The listing builds one solid part. Answer for the finished solid, in the listing's coordinates (mm). A direction names the side the tool comes from. Round coordinates to 2 decimals unless told otherwise and drop trailing zeros. Write each loop counter-clockwise with the first axis right and the second up, starting at its lowest first coordinate (ties: lowest second). Pieces come first, ordered by that corner, then holes.
(1) Find the intervals of material crossed by probe 1 along X at (y, z) = (10.8, 0); probe 2 along Y at (x, z) = (0, 11.75) (3 decimals); probe 3 along X at (y, z) = (7, 2.5), in increasing order.
(2) A cutting plane is placed at C-C, the plane x = 17.5. Give the vertices of the cut face in (y, z).
(3) For faces 4 (the face through (0, 6, -20.41)), 5 (the face through (-0.116, 2.827, 7.888)), 6 (the face through (0, 9, -18)), determine the directions among +Z, -Z, +X, -X, +Y, -Y from which every point of the face is accessible in a straight line to the end or side of a thin tool.
(4) The mould has two halves that part along Y. Classify faces 1 (the face through (-2.93, 5.92, -20.26)), 2 (the face through (0, 8.75, 8)), 3 (the face through (0, 12, 0)): +Y half, -Y half, draft (parallel to the pull), parting line (faces both ways), or undercut.
(5) A cutting plane is placed at B-B, the plane y = 11.25. Give the vertices of the cut face in (x, z).
(6) Each of these flat-tipped pins is pushed along its axis until it touches: pin 1 Ø1.5 at (x, z) = (-17, -0.5) entering from +Y; pin 2 Ø1 at (y, z) = (3.5, -7.5) entering from -X; pin 3 Ø1.5 at (x, y) = (5.5, 10.5) entering from +Z. Where does it stop, or does it pass through?
from build123d import *

# Parameters (mm, degrees)
BOSS_EXTRUDE1_DEPTH = 12
SKETCH3_R           = 1.5
CUT_EXTRUDE1_DEPTH  = 3
CUT_EXTRUDE2_DEPTH  = 25.4
FILLET1_R           = 2


with BuildPart() as part:
    # Sketch1 → Boss-Extrude1 (new body)
    with BuildSketch(Plane(origin=(0, 0, 0), x_dir=(1, 0, 0), z_dir=(0, 1, 0))):
        Polygon((-3, -20.41), (3, -20.41), (20.41, -3), (20.41, 3), (3, 20.41), (-3, 20.41), (-20.41, 3), (-20.41, -3), align=None)
    extrude(amount=BOSS_EXTRUDE1_DEPTH)

    # Sketch3 → Cut-Extrude1 (cut)
    with BuildSketch(Plane(origin=(0, 12, 0), x_dir=(1, 0, 0), z_dir=(0, 1, 0))):
        with Locations(Location((17.5, 0, 0), (0, 0, 270))):
            Circle(SKETCH3_R)
        with Locations(Location((0, -17.5, 0), (0, 0, 270))):
            Circle(SKETCH3_R)
        with Locations(Location((-17.5, 0, 0), (0, 0, 270))):
            Circle(SKETCH3_R)
        with Locations(Location((0, 17.5, 0), (0, 0, 270))):
            Circle(SKETCH3_R)
    extrude(amount=-CUT_EXTRUDE1_DEPTH, mode=Mode.SUBTRACT)

    # Sketch2 → Cut-Extrude2 (cut)
    with BuildSketch(Plane.XY.offset(20.41)):
        with BuildLine():
            Line((1.5875, 8.749630657), (-1.5875, 8.749630657))
            ThreePointArc((-1.5875, 8.749630657), (0, 2.825), (1.5875, 8.749630657))
        make_face()
    extrude(amount=-CUT_EXTRUDE2_DEPTH, mode=Mode.SUBTRACT)

    # Fillet1
    # the kernel refuses this fillet: 2 mm, written as the material it takes off along each edge
    with BuildSketch(Plane(origin=(20.41, -2.071067812, -3), x_dir=(0, 0, 1), z_dir=(0, 1, 0)), Plane(origin=(20.41, -2.071067812, 3), x_dir=(-0.7071067811865513, 0, 0.7071067811865438), z_dir=(0, 1, 0)), Plane(origin=(-20.41, -2.071067812, -3), x_dir=(0.7071067811865451, 0, -0.70710678118655), z_dir=(0, 1, 0)), Plane(origin=(-3, -2.071067812, -20.41), x_dir=(1, 0, 0), z_dir=(0, 1, 0)), Plane(origin=(3, -2.071067812, -20.41), x_dir=(0.7071067811865518, 0, 0.7071067811865432), z_dir=(0, 1, 0))) as fillet1_piece_1:
        with BuildLine():
            CenterArc((FILLET1_R * 0.414213562373, -FILLET1_R), FILLET1_R, 90, 45)
            Line((-FILLET1_R * 0.292893218813, -FILLET1_R * 0.292893218813), (0, 0))
            Line((0, 0), (FILLET1_R * 0.414213562373, 0))
        make_face()
    extrude(amount=16.142135624, mode=Mode.SUBTRACT)
    with BuildSketch(Plane(origin=(3, 4.968463332, 20.41), x_dir=(0.7071067811865491, 0, -0.7071067811865459), z_dir=(0, 1, 0)), Plane(origin=(-3, -2.071067812, 20.41), x_dir=(1, 0, 0), z_dir=(0, 1, 0))) as fillet1_piece_2:
        with BuildLine():
            CenterArc((FILLET1_R * 0.414213562373, FILLET1_R), FILLET1_R, 225, 45)
            Line((-FILLET1_R * 0.292893218813, FILLET1_R * 0.292893218813), (0, 0))
            Line((0, 0), (FILLET1_R * 0.414213562373, 0))
        make_face()
    extrude(amount=9.102604479, mode=Mode.SUBTRACT)
    with BuildSketch(Plane(origin=(-3, 4.968463332, 20.41), x_dir=(-0.7071067811865411, 0, -0.707106781186554), z_dir=(0, 1, 0)), Plane(origin=(3, -2.071067812, 20.41), x_dir=(-1, 0, 0), z_dir=(0, 1, 0))) as fillet1_piece_3:
        with BuildLine():
            CenterArc((FILLET1_R * 0.414213562373, -FILLET1_R), FILLET1_R, 90, 45)
            Line((-FILLET1_R * 0.292893218813, -FILLET1_R * 0.292893218813), (0, 0))
            Line((0, 0), (FILLET1_R * 0.414213562373, 0))
        make_face()
    extrude(amount=9.102604479, mode=Mode.SUBTRACT)
    with BuildSketch(Plane(origin=(-20.41, -2.071067812, 3), x_dir=(0.7071067811865429, 0, 0.7071067811865521), z_dir=(0, 1, 0))) as fillet1_piece_4:
        with BuildLine():
            CenterArc((FILLET1_R * 0.414213562373, FILLET1_R), FILLET1_R, 225, 45)
            Line((-FILLET1_R * 0.292893218813, FILLET1_R * 0.292893218813), (0, 0))
            Line((0, 0), (FILLET1_R * 0.414213562373, 0))
        make_face()
    extrude(amount=16.142135624, mode=Mode.SUBTRACT)


solid = part.part
Solutions:
1. probe 1: x = -20.41 to -19, -16 to 16, 19 to 20.41
1. probe 2: y = 0 to 2.825, 8.75 to 12
1. probe 3: x = -20.38 to -3.01, 3.01 to 20.38
2. outline: (0, -5.91) - (12, -5.91) - (12, -1.5) - (9, -1.5) - (9, 1.5) - (12, 1.5) - (12, 5.91) - (0, 5.91) - close
3. face 4: -Z, +X, -X, +Y, -Y
3. face 5: +Z
3. face 6: +Y
4. face 1: draft
4. face 2: undercut
4. face 3: +Y half
5. outline: (-20.41, -2.17) arc R2 ccw to (-19.82, -3.59) - (-3.59, -19.82) arc R2 ccw to (-2.17, -20.41) - (2.17, -20.41) arc R2 ccw to (3.59, -19.82) - (19.82, -3.59) arc R2 ccw to (20.41, -2.17) - (20.41, 2.17) arc R2 ccw to (19.82, 3.59) - (3.59, 19.82) arc R2 ccw to (2.17, 20.41) - (-2.17, 20.41) arc R2 ccw to (-3.59, 19.82) - (-19.82, 3.59) arc R2 ccw to (-20.41, 2.17) - close; hole circle Ø3 at (-17.5, 0); hole circle Ø3 at (0, -17.5); hole circle Ø3 at (0, 17.5); hole circle Ø3 at (17.5, 0)
6. pin 1: stops at y = 9
6. pin 2: stops at x = -16.41
6. pin 3: stops at z = 18.66
